For this review, take the finished solid that the model builds, in its own axes (mm). A direction names the side the tool comes from. Give positions to 0.01 mm unless a question says otherwise; leave off trailing zeros. Loops run counter-clockwise (first coordinate to the right, second up) from the corner with the lowest first, then second, coordinate; pieces in that order, holes last. Notation, with made-up numbers: (31.25, 34.5) - (58.25, 34.5) arc R19 cw to (58.25, 39.5) - close; hole circle Ø9 at (-9, 18). An arc over 180 degrees is marked (long way). Answer as CSV lines item,"result".
from build123d import *

# Parameters (mm, degrees)
BOSS_EXTRUDE1_DEPTH   = 15
SKETCH5_R             = 2
CUT_EXTRUDE3_DEPTH    = 15
D_GAGEMENT_M41_D      = 4.5
D_GAGEMENT_M41_DEPTH  = 12
TROU_TARAUD_M41_D     = 3.3
TROU_TARAUD_M41_DEPTH = 12


with BuildPart() as part:
    # Sketch1 → Boss-Extrude1 (new body)
    with BuildSketch(Plane.XY):
        with BuildLine():
            Line((-26, 0), (-26, -40))
            Line((-26, -40), (-38, -40))
            Line((-38, -40), (-38, -50))
            Line((-38, -50), (12, -50))
            Line((12, -50), (12, -40))
            Line((12, -40), (0, -40))
            Line((0, -40), (0, 0))
            Line((0, 0), (-12, 0))
            Line((-12, 0), (-12, -13.07179677))
            ThreePointArc((-12, -13.07179677), (-13, -27), (-14, -13.07179677))
            Line((-14, -13.07179677), (-14, 0))
            Line((-14, 0), (-26, 0))
        make_face()
    extrude(amount=BOSS_EXTRUDE1_DEPTH)

    # Sketch5 → Cut-Extrude3 (cut)
    with BuildSketch(Plane(origin=(0, -40, 0), x_dir=(1, 0, 0), z_dir=(0, 1, 0))):
        with Locations((6, -7.5)):
            Circle(SKETCH5_R)
        with Locations((-32, -7.5)):
            Circle(SKETCH5_R)
    extrude(amount=-CUT_EXTRUDE3_DEPTH, mode=Mode.SUBTRACT)

    # Dégagement M41
    with Locations(Plane.ZY.offset(26)):
        with Locations((7.569852971, -7)):
            Hole(D_GAGEMENT_M41_D / 2, depth=D_GAGEMENT_M41_DEPTH)

    # Trou taraudé M41
    with Locations(Plane(origin=(0, 0, 0), x_dir=(0, 0, -1), z_dir=(1, 0, 0))):
        with Locations((-7.5, -7)):
            Hole(TROU_TARAUD_M41_D / 2, depth=TROU_TARAUD_M41_DEPTH)


solid = part.part
1) Consider section A-A on x = 6. Write out the cut boundary in (y, z).
From the geometry:
outline,"(-50, 0) - (-40, 0) - (-40, 5.5) - (-50, 5.5) - close; (-50, 9.5) - (-40, 9.5) - (-40, 15) - (-50, 15) - close"
2) Consider section B-B on x = -8.5. Write out the cut boundary in (y, z).
From the geometry:
outline,"(-50, 0) - (-25.36, 0) - (-25.36, 15) - (-50, 15) - close; (-14.64, 0) - (0, 0) - (0, 15) - (-14.64, 15) - close; hole circle Ø3.3 at (-7, 7.5)"
3) Consider section D-D on z = 7.5. Write out the cut boundary in (x, y).
From the geometry:
outline,"(-38, -50) - (-34, -50) - (-34, -40) - (-38, -40) - close; (-30, -50) - (4, -50) - (4, -40) - (0, -40) - (0, -8.65) - (-12, -8.65) - (-12, -13.07) arc R7 cw (long way) to (-14, -13.07) - (-14, -9.25) - (-26, -9.25) - (-26, -40) - (-30, -40) - close; (-26, -4.75) - (-14, -4.75) - (-14, 0) - (-26, 0) - close; (-12, -5.35) - (0, -5.35) - (0, 0) - (-12, 0) - close; (8, -50) - (12, -50) - (12, -40) - (8, -40) - close"
4) Machinability: for faces 1 (the flat face through (7.4, -40, 5.7)), 2 (the flat face through (-30.6, -40, 5.7)), 3 (the flat face through (-14, -5, 6)), which of the approach directions +Z, -Z, +X, -X, +Y, -Y give a long, thin tool a straight path to every point of the face, cutting with its end or side? Answer none if there is none.
From the geometry:
face 1,"+Z, -Z, +X, +Y"
face 2,"+Z, -Z, -X, +Y"
face 3,"+Z, -Z, +Y"
5) Draft analysis for pull direction Z (two halves, no side actions). For faces 4 (the flat face through (-13, -30, 15)), 5 (the cylindrical face through (-6.08, -8, 6.19)), 6 (the cylindrical face through (-13, -27, 7)), state which applies: pulls with the +Z half, pulls with the -Z half, needs draft (parallel to the pull), parting line crosses it, or undercut.
From the geometry:
face 4,"pulls with the +Z half"
face 5,"undercut"
face 6,"needs draft"
6) Wall thickness on line 1 (Y direction, x = -5, z = 7.5); line 2 (X direction, y = -4, z = 9.5); line 3 (Z direction, x = -32, y = -44.25): over which ranges is each line inside the solid? List them lowest first. Write a range as from..to.
From the geometry:
line 1,"y = -50..-8.65, -5.35..0"
line 2,"x = -26..-14, -12..0"
line 3,"z = 0..5.5, 9.5..15"
7) Consider section C-C on y = -11.5. Write out the cut boundary in (x, z), and give its area (3 significant figures).
From the geometry:
outline,"(-26, 0) - (-14, 0) - (-14, 15) - (-26, 15) - close; (-12, 0) - (0, 0) - (0, 15) - (-12, 15) - close"
area,"360 mm^2"
8) Insertion check: P1, Ø6, axis at y = -25.5, z = 3.5, coming from the -X side; P2, Ø6, axis at y = -5, z = 12, coming from the +X side; P3, Ø6, axis at x = -34.5, z = 9.5, coming from the +Y side. Each pin has a flat end and moves straight along its axis. Give the tip position at first contact, or say it passes through.
From the geometry:
P1,"stops at x = -26"
P2,"stops at x = 0"
P3,"stops at y = -40"
